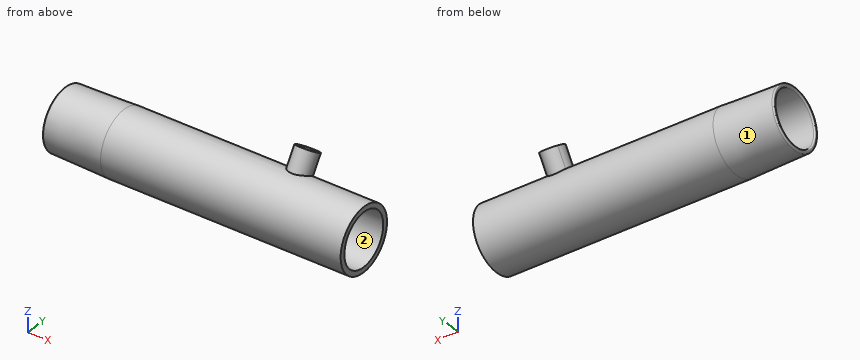
```python
from build123d import *

# Parameters (mm, degrees)
BOSS_EXTRUDE1_START = -21
SKETCH2_R           = 10.322343774
SKETCH2_R_2         = 9.5
BOSS_EXTRUDE1_DEPTH = 21
FILLET1_R           = 0.5
SKETCH3_R           = 11.335
SKETCH3_R_2         = 9.5
BOSS_EXTRUDE2_DEPTH = 85
BOSS_EXTRUDE3_START = 9.334999999
BOSS_EXTRUDE3_DEPTH = 8.999999999
SKETCH5_R           = 3.050000003
CUT_EXTRUDE1_DEPTH  = 11


# Read off the part's stored shape, not the designer's step: Boss-Extrude3
with BuildPart() as part:
    # Sketch1 → Revolve1 (revolve)
    with BuildSketch(Plane.XY, mode=Mode.PRIVATE) as revolve1_sk:
        with BuildLine():
            Line((6, 11.335), (-14.512496096, 10.822187598))
            ThreePointArc((-14.512496096, 10.822187598), (-14.857944163, 10.671451174), (-15, 10.322343774))
            Line((-15, 10.322343774), (6, 10.322343774))
            Line((6, 10.322343774), (6, 11.335))
        make_face()
    revolve(revolve1_sk.sketch.rotate(Axis((-15.624243475, 0, 0), (1, 0, 0)), 90), axis=Axis((-15.624243475, 0, 0), (1, 0, 0)))

    # Sketch2 → Boss-Extrude1 (add)
    with BuildSketch(Plane(origin=(6, 0, 0), x_dir=(0, 0, -1), z_dir=(1, 0, 0)).offset(BOSS_EXTRUDE1_START)):
        Circle(SKETCH2_R)
        Circle(SKETCH2_R_2, mode=Mode.SUBTRACT)
    extrude(amount=BOSS_EXTRUDE1_DEPTH)

    # Fillet1
    fillet1_edges = [part.edges().sort_by_distance(p)[0] for p in [
        (-15, 0, 9.5),
    ]]
    fillet(fillet1_edges, radius=FILLET1_R)

    # Sketch3 → Boss-Extrude2 (add)
    with BuildSketch(Plane(origin=(6, 0, 0), x_dir=(0, 0, -1), z_dir=(1, 0, 0))):
        Circle(SKETCH3_R)
        Circle(SKETCH3_R_2, mode=Mode.SUBTRACT)
    extrude(amount=BOSS_EXTRUDE2_DEPTH)

    # Boss-Extrude3 outline → Boss-Extrude3 (add)
    with BuildSketch(Plane(origin=(0, 0, 0), x_dir=(1, 0, 0), z_dir=(0, 0.5487408887134131, 0.8359924862425581)).offset(BOSS_EXTRUDE3_START)):
        with BuildLine():
            ThreePointArc((60.34828113, -1.762888304), (68.110256528, -1.132677071), (60.881070562, 1.762888255))
            ThreePointArc((60.881070562, 1.762888255), (60.200061526, 0.062653443), (60.34828113, -1.762888304))
        make_face()
    extrude(amount=BOSS_EXTRUDE3_DEPTH)

    # Sketch5 → Cut-Extrude1 (cut)
    with BuildSketch(Plane(origin=(0, 10.061164202, 15.32792223), x_dir=(1, 0, 0), z_dir=(1.7486012637846212e-15, 0.5487408891490924, 0.8359924859565806))):
        with Locations(Location((64.155159027, -0.535011823, 0), (0, 0, 270))):
            Circle(SKETCH5_R)
    extrude(amount=-CUT_EXTRUDE1_DEPTH, mode=Mode.SUBTRACT)


solid = part.part
```
Could you check a few things on this model? Use its own coordinates, in mm. Face numbers are marked on the shaded views. Coordinates: 2 decimals unless noted, no trailing zeros. Write each loop counter-clockwise with the first axis right and the second up, starting at its lowest first coordinate (ties: lowest second). Pieces come first, ordered by that corner, then holes. Notation, with made-up numbers: (-5.75, -16) - (37.25, -16) arc R30 ccw to (37.25, 23) - close; hole circle Ø1 at (40.25, 4.5). An arc over 180 degrees is marked (long way). Use a Markdown table: item, result.
Q1. Please list where these lines run through material, in increasing order: L1, parallel to Y at x = 25, z = 0 (3 decimals); L2, parallel to Y at x = 2, z = 7; L3, parallel to Z at x = 31.5, y = 4.5.
Geometry check:
| item | result |
|---|---|
| L1 | y = -11.335 to -9.5, 9.5 to 11.335 |
| L2 | y = -8.79 to -6.42, 6.42 to 8.79 |
| L3 | z = -10.4 to -8.37, 8.37 to 10.4 |
Q2. Thinking about a two-plate mould opening in Y: for the marked faces 1 and 2, which applies, +Y half, -Y half, draft (parallel to the pull), parting line (faces both ways), or undercut?
Geometry check:
| item | result |
|---|---|
| face 1 | parting line |
| face 2 | undercut |
Q3. I'm going to push flat-ended pins straight in: pin 1 Ø4 at (x, z) = (75.5, 4.5) entering from -Y; pin 2 Ø10 at (x, z) = (31.5, 9) entering from -Y; pin 3 Ø10 at (x, z) = (15, 7) entering from -Y; pin 4 Ø2 at (y, z) = (-2.5, 12.5) entering from -X. Where does each tip first touch, or does it pass through?
Geometry check:
| item | result |
|---|---|
| pin 1 | stops at y = -11.06 |
| pin 2 | stops at y = -10.61 |
| pin 3 | stops at y = -11.16 |
| pin 4 | passes through |
Q4. Imagine slicing it at C-C (x = 37). List the corners of the cut face in (y, z) for me (3 decimals).
Geometry check:
| item | result |
|---|---|
| outline | circle Ø22.67 at (0, 0); hole circle Ø19 at (0, 0) |
